from build123d import *

# Parameters (mm, degrees)
EXTRUDE_1_DEPTH     = 5
SKETCH_2_W          = 20
SKETCH_2_H          = 20.2
CUT_EXTRUDE_1_DEPTH = 6
SKETCH_3_R          = 1.15
EXTRUDE_2_DEPTH     = 6
CHAMFER_1_SIZE      = 5
SKETCH_4_R          = 1.6
CUT_EXTRUDE_2_DEPTH = 32
SKETCH_5_R          = 2.75
CUT_EXTRUDE_3_DEPTH = 6


with BuildPart() as part:
    # 草图1 → 凸台-拉伸1 (new body, symmetric)
    with BuildSketch(Plane(origin=(0, 0, 0), x_dir=(0, 0, -1), z_dir=(1, 0, 0))):
        Polygon((0, 0), (15, 0), (15, 23), (35, 23), (35, 31), (10, 31), (10, 4), (0, 4), align=None)
    extrude(amount=EXTRUDE_1_DEPTH, both=True)

    # 草图2 → 切除-拉伸1 (cut)
    with BuildSketch(Plane(origin=(0, 31, 0), x_dir=(1, 0, 0), z_dir=(0, 1, 0))):
        with Locations((5, 22.5)):
            Rectangle(SKETCH_2_W, SKETCH_2_H)
    extrude(amount=-CUT_EXTRUDE_1_DEPTH, mode=Mode.SUBTRACT)

    # 草图3 → 凸台-拉伸2 (add)
    with BuildSketch(Plane(origin=(0, 25, 0), x_dir=(1, 0, 0), z_dir=(0, 1, 0))):
        with Locations((2, 27.25)):
            Circle(SKETCH_3_R)
        with Locations((2, 17.75)):
            Circle(SKETCH_3_R)
    extrude(amount=EXTRUDE_2_DEPTH)

    # 倒角1
    chamfer_1_edges = [part.edges().sort_by_distance(p)[0] for p in [
        (0, 4, -10),
        (0, 23, -15),
    ]]
    chamfer(chamfer_1_edges, length=CHAMFER_1_SIZE)

    # 草图4 → 切除-拉伸2 (cut, through all)
    with BuildSketch(Plane.XZ):
        with Locations((0, -6)):
            Circle(SKETCH_4_R)
    extrude(amount=-CUT_EXTRUDE_2_DEPTH, mode=Mode.SUBTRACT)

    # 草图5 → 切除-拉伸3 (cut)
    with BuildSketch(Plane(origin=(0, 4, 0), x_dir=(1, 0, 0), z_dir=(0, 1, 0))):
        with Locations((0, 6)):
            Circle(SKETCH_5_R)
    extrude(amount=CUT_EXTRUDE_3_DEPTH, mode=Mode.SUBTRACT)


solid = part.part
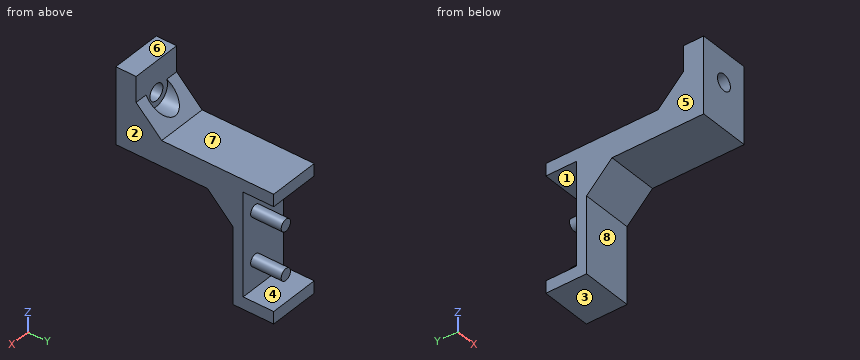
Design review of the part built by this model. Coordinates are the model's own, in mm. Face numbers are marked on the shaded views. A direction names the side the tool comes from. Round coordinates to 2 decimals unless told otherwise and drop trailing zeros. Loops run counter-clockwise (first coordinate to the right, second up) from the corner with the lowest first, then second, coordinate; pieces in that order, holes last. Notation, with made-up numbers: (62.5, 23) - (98.5, 23) arc R28 ccw to (98.5, 53) - close; hole circle Ø7 at (61, 17). An arc over 180 degrees is marked (long way). One line per question, with ' | ' between items.
1. We need section B-B, the plane x = 0. State the section outline as (y, z) points, and give its area (3 significant figures).
Results are:
outline: (0, -15) - (18, -15) - (23, -20) - (23, -35) - (31, -35) - (31, -32.6) - (25, -32.6) - (25, -12.4) - (31, -12.4) - (31, -10) - (9, -10) - (7.75, -8.75) - (4, -8.75) - (4, -7.6) - (0, -7.6) - close; (0, -4.4) - (4, -4.4) - (4, 0) - (0, 0) - close | area: 239 mm²
2. We need section A-A, the plane z = -6. State the section outline as (x, y) points, and give its area (3 significant figures).
Results are:
outline: (-5, 0) - (-1.6, 0) - (-1.6, 4) - (-2.75, 4) - (-2.75, 5) - (-5, 5) - close; (1.6, 0) - (5, 0) - (5, 5) - (2.75, 5) - (2.75, 4) - (1.6, 4) - close | area: 31.7 mm²
3. We need section D-D, the plane z = -27.25. State the section outline as (x, y) points.
Results are:
outline: (-5, 23) - (5, 23) - (5, 25) - (3.15, 25) - (3.15, 31) - (0.85, 31) - (0.85, 25) - (-5, 25) - close
4. For L1, parallel to Z at x = 0, y = 2.75; L2, parallel to Z at x = -3.25, y = 25.5; L3, parallel to Z at x = 0, y = 5.2, list the stretches that pass through material, from the lowest coordinate up. Write a range as [from, to].
Results are:
L1: z = [-15, -7.6], [-4.4, 0] | L2: z = [-35, -32.6], [-12.4, -10] | L3: z = [-15, -8.75]
5. Clearance check with flat-ended pins moving along their axes: P1, Ø5, axis at x = -1, z = -28, coming from the -Y side; P2, Ø2, axis at y = 8.5, z = -7.5, coming from the +X side (3 decimals); P3, Ø1.5, axis at y = 28, z = -19, coming from the +X side; P4, Ø5, axis at x = 0.5, y = 7.5, coming from the -Z side. State where each tip first meets the part, or that it passes through.
Results are:
P1: stops at y = 23 | P2: passes through | P3: stops at x = 3.04 | P4: stops at z = -15
6. For the marked faces 4, 5, 6, 7 and 8, list the 3-axis set-ups (+Z, -Z, +X, -X, +Y, -Y) from which the entire face can be reached by the end or side of a thin tool; tool diameter is ignored.
Results are:
face 4: +X, -X, +Y | face 5: +Z, -Z, -X, +Y, -Y | face 6: +Z, +X, -X, +Y, -Y | face 7: +Z, +X, -X, +Y | face 8: -Z, +X, -X, -Y
7. Draft analysis for pull direction Z (two halves, no side actions). For the marked faces 1, 2 and 3, state which applies: released by +Z, released by -Z, zero draft, split by the parting line, or undercut.
Results are:
face 1: undercut | face 2: zero draft | face 3: released by -Z
8. We need section C-C, the plane x = 3.75. State the section outline as (y, z) points, and give its area (3 significant figures).
Results are:
outline: (0, -15) - (18, -15) - (23, -20) - (23, -35) - (31, -35) - (31, -32.6) - (25, -32.6) - (25, -12.4) - (31, -12.4) - (31, -10) - (9, -10) - (4, -5) - (4, 0) - (0, 0) - close | area: 259 mm²
